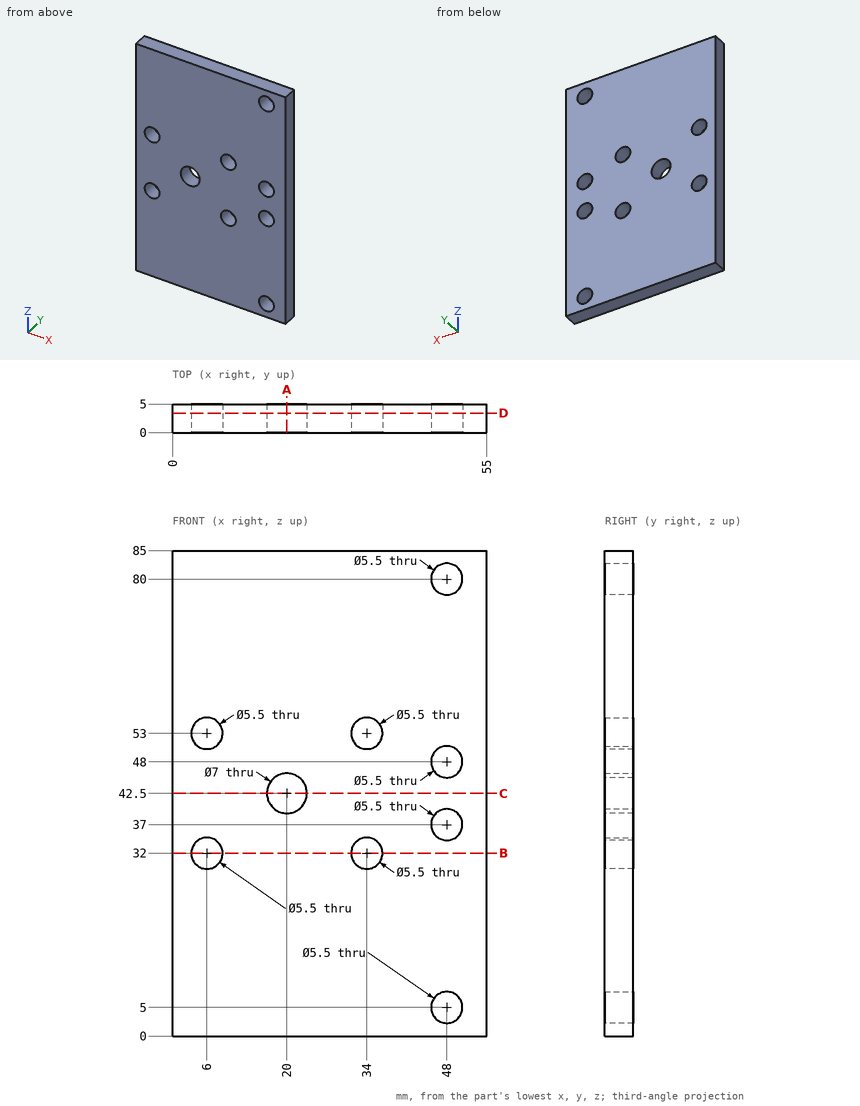
Verification items for this drawing (mm, ordinates from the low corner). Give positions to 0.01 mm unless a question says otherwise; leave off trailing zeros. Loops run counter-clockwise (first coordinate to the right, second up) from the corner with the lowest first, then second, coordinate; pieces in that order, holes last. Notation, with made-up numbers: M 7.25,-21.75 L 23.25,-21.75 A19 cw 23.25,6.25 Z; hole C 47.5,-38 d4. An arc over 180 degrees is marked long. Answer as CSV lines item,"result".
Item 1: Cross-section at D-D on y = 3.4. Count the separate pieces of the cut face and the enclosed holes in it, and give its area (3 significant figures).
Values:
separate pieces,"1"
enclosed holes,"9"
area,"4,450 mm²"
Item 2: Cross-section at B-B on z = 32. Record the cut outline in (x, y), and give its area (3 significant figures).
Values:
outline,"M 0,0 L 3.25,0 L 3.25,5 L 0,5 Z; M 8.75,0 L 31.25,0 L 31.25,5 L 8.75,5 Z; M 36.75,0 L 55,0 L 55,5 L 36.75,5 Z"
area,"220 mm²"
Item 3: Cross-section at C-C on z = 42.5. Record the cut outline in (x, y).
Values:
outline,"M 0,0 L 16.5,0 L 16.5,5 L 0,5 Z; M 23.5,0 L 55,0 L 55,5 L 23.5,5 Z"
Item 4: Cross-section at A-A on x = 20. Record the cut outline in (y, z).
Values:
outline,"M 0,0 L 5,0 L 5,39 L 0,39 Z; M 0,46 L 5,46 L 5,85 L 0,85 Z"
Item 5: Depth check by flat-ended pin: P1, Ø8, axis at x = 20, z = 42.5, coming from the +Y side. Enter the tip coordinate at first touch or a pass-through.
Values:
P1,"stops at y = 5"
Item 6: Material ranges on line 1 (X direction, y = 3.05, z = 53); line 2 (Z direction, x = 6, y = 0.3); line 3 (Z direction, x = 8, y = 2.55), recorded low to high.
Values:
line 1,"x = 0 to 3.25, 8.75 to 31.25, 36.75 to 55"
line 2,"z = 0 to 29.25, 34.75 to 50.25, 55.75 to 85"
line 3,"z = 0 to 30.11, 33.89 to 51.11, 54.89 to 85"
